Verification items for this drawing (mm, ordinates from the low corner). Round coordinates to 2 decimals unless told otherwise and drop trailing zeros. Order: outer loops, then holes, each group sorted by start corner. A loop starts at its lowest first (then second) coordinate and runs counter-clockwise, first axis right, second up.
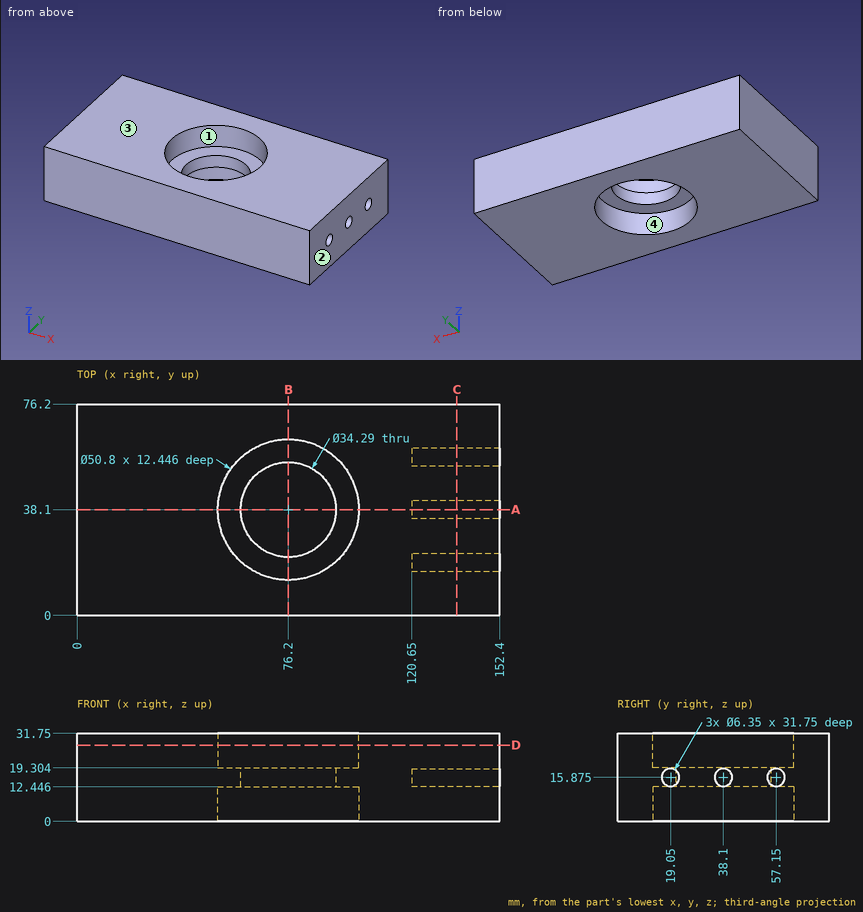
Item 1: Sectioned sample at A-A (y = 38.1). Record the cut outline in (x, z) (3 decimals).
Answer:
outline: (0, 0) - (50.8, 0) - (50.8, 12.446) - (59.055, 12.446) - (59.055, 19.304) - (50.8, 19.304) - (50.8, 31.75) - (0, 31.75) - close; (93.345, 12.446) - (101.6, 12.446) - (101.6, 0) - (152.4, 0) - (152.4, 12.7) - (120.65, 12.7) - (120.65, 19.05) - (152.4, 19.05) - (152.4, 31.75) - (101.6, 31.75) - (101.6, 19.304) - (93.345, 19.304) - close
Item 2: Sectioned sample at C-C (x = 137). Record the cut outline in (y, z) (3 decimals), and give its area (3 significant figures).
Answer:
outline: (0, 0) - (76.2, 0) - (76.2, 31.75) - (0, 31.75) - close; hole circle Ø6.35 at (19.05, 15.875); hole circle Ø6.35 at (38.1, 15.875); hole circle Ø6.35 at (57.15, 15.875)
area: 2,320 mm2
Item 3: Sectioned sample at D-D (z = 27.5). Record the cut outline in (x, y).
Answer:
outline: (0, 0) - (152.4, 0) - (152.4, 76.2) - (0, 76.2) - close; hole circle Ø50.8 at (76.2, 38.1)
Item 4: Scan lines: line 1 along Z through (x, y) = (130, 19); line 2 along Y through (x, z) = (76, 15); line 3 along Y through (x, z) = (76, 26). Record each from-to range of solid material in increasing order.
Answer:
line 1: z = 0 to 12.7, 19.05 to 31.75
line 2: y = 0 to 20.96, 55.24 to 76.2
line 3: y = 0 to 12.7, 63.5 to 76.2
Item 5: Sectioned sample at B-B (x = 76.2). Record the cut outline in (y, z) (3 decimals).
Answer:
outline: (0, 0) - (12.7, 0) - (12.7, 12.446) - (20.955, 12.446) - (20.955, 19.304) - (12.7, 19.304) - (12.7, 31.75) - (0, 31.75) - close; (55.245, 12.446) - (63.5, 12.446) - (63.5, 0) - (76.2, 0) - (76.2, 31.75) - (63.5, 31.75) - (63.5, 19.304) - (55.245, 19.304) - close
Item 6: Go/stop test with flat-tipped pins: P1, Ø5, axis at y = 19.05, z = 15.875, coming from the +X side; P2, Ø15, axis at x = 73.5, y = 40.5, coming from the -Z side; P3, Ø5, axis at x = 91, y = 32.5, coming from the +Z side. Record where each tip stops, or that it passes through.
Answer:
P1: stops at x = 120.65
P2: passes through
P3: stops at z = 19.3
Item 7: Release check for a two-part mould opening along X. For the marked faces 1, 2, 3 and 4 record: released by +X, released by -X, zero draft, split by the parting line, or undercut.
Answer:
face 1: undercut
face 2: released by +X
face 3: zero draft
face 4: undercut
